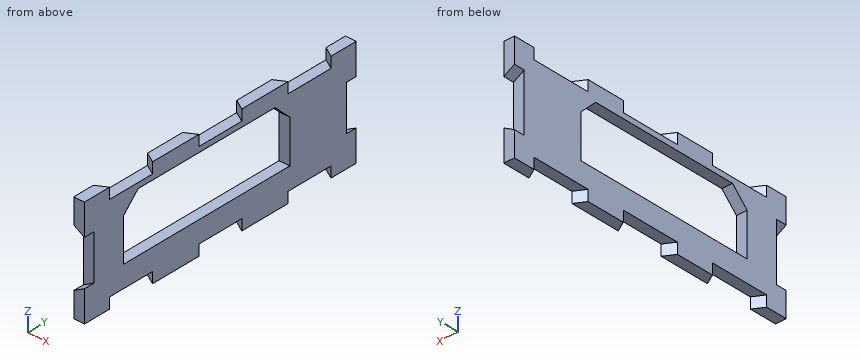
from build123d import *

# Parameters (mm, degrees)
SKETCH2_W           = 139
SKETCH2_H           = 50
BOSS_EXTRUDE1_DEPTH = 5
CUT_EXTRUDE1_DEPTH  = 5
CUT_EXTRUDE2_START  = -45
CUT_EXTRUDE2_DEPTH  = 5
CUT_EXTRUDE3_DEPTH  = 5
CUT_EXTRUDE5_START  = -134
CUT_EXTRUDE5_DEPTH  = 5
CUT_EXTRUDE6_DEPTH  = 5


with BuildPart() as part:
    # Sketch2 → Boss-Extrude1 (new body)
    with BuildSketch(Plane.YZ):
        Rectangle(SKETCH2_W, SKETCH2_H)
    extrude(amount=BOSS_EXTRUDE1_DEPTH)

    # Sketch3 → Cut-Extrude1 (cut)
    with BuildSketch(Plane(origin=(0, 0, -25), x_dir=(1, 0, 0), z_dir=(0, 0, -1))):
        Polygon((0, 31.787187079), (0, 59.5), (24, 45.643593539), align=None)
        Polygon((0, -13.856406461), (0, 13.856406461), (24, 0), align=None)
        Polygon((0, -59.5), (0, -31.787187079), (24, -45.643593539), align=None)
    extrude(amount=-CUT_EXTRUDE1_DEPTH, mode=Mode.SUBTRACT)

    # Sketch3<3> → Cut-Extrude2 (cut)
    with BuildSketch(Plane(origin=(0, 0, -25), x_dir=(1, 0, 0), z_dir=(0, 0, -1)).offset(CUT_EXTRUDE2_START)):
        Polygon((0, 31.787187079), (0, 59.5), (24, 45.643593539), align=None)
        Polygon((0, -13.856406461), (0, 13.856406461), (24, 0), align=None)
        Polygon((0, -59.5), (0, -31.787187079), (24, -45.643593539), align=None)
    extrude(amount=-CUT_EXTRUDE2_DEPTH, mode=Mode.SUBTRACT)

    # Sketch6 → Cut-Extrude3 (cut)
    with BuildSketch(Plane(origin=(0, 69.5, 0), x_dir=(-1, 0, 0), z_dir=(0, 1, 0))):
        Polygon((0, 13.423393759), (0, -13.423393759), (-23.25, 0), align=None)
    extrude(amount=-CUT_EXTRUDE3_DEPTH, mode=Mode.SUBTRACT)

    # Sketch6<3> → Cut-Extrude5 (cut)
    with BuildSketch(Plane(origin=(0, 69.5, 0), x_dir=(-1, 0, 0), z_dir=(0, 1, 0)).offset(CUT_EXTRUDE5_START)):
        Polygon((0, 13.423393759), (0, -13.423393759), (-23.25, 0), align=None)
    extrude(amount=-CUT_EXTRUDE5_DEPTH, mode=Mode.SUBTRACT)

    # Sketch4 → Cut-Extrude6 (cut)
    with BuildSketch(Plane(origin=(0, 0, 0), x_dir=(0, -1, 0), z_dir=(-1, 0, 0))):
        Polygon((-35.5, -10), (49.5, -10), (49.5, 10), (42, 17.5), (-28, 17.5), (-35.5, 10), align=None)
    extrude(amount=-CUT_EXTRUDE6_DEPTH, mode=Mode.SUBTRACT)


solid = part.part
The model under review builds one solid part; all positions refer to its coordinate system, in mm. Round coordinates to 2 decimals unless told otherwise and drop trailing zeros. Loops run counter-clockwise (first coordinate to the right, second up) from the corner with the lowest first, then second, coordinate; pieces in that order, holes last. Notation, with made-up numbers: (-30.75, -26.5) -> (-5.75, -26.5) arc R25 cw to (-5.75, -14.5) -> close; hole circle Ø11 at (28.5, -19). An arc over 180 degrees is marked (long way). Write item = value, one per line. Start each with the question number.
Item 1: Take a section at B-B on y = -40. Give the boundary of the cut face in (x, z), plus the area to 3 significant figures.
Item 2: Insertion check: pin 1 (2.5 mm diameter, centred on x = 1.5, y = -6, fed in from -Z); pin 2 (2.5 mm diameter, centred on x = 2.5, z = -2.5, fed in from -Y); pin 3 (1.5 mm diameter, centred on x = 3.5, y = -43.5, fed in from +Z). Each pin has a flat end and moves straight along its axis. Give the tip position at first contact, or say it passes through.
Item 3: Take a section at D-D on z = -12. Give the boundary of the cut face in (x, y).
Item 4: Take a section at C-C on y = 50. Give the boundary of the cut face in (x, z).
Item 5: To check wall thickness, follow L1, parallel to Y at x = 4, z = 5; L2, parallel to Z at x = 2.65, y = -19; L3, parallel to Z at x = 3.6, y = -1. State the ranges of each line that lie inside material, in increasing order.
Item 6: Take a section at A-A on z = -3. Give the boundary of the cut face in (x, y), plus the area to 3 significant figures.
Result:
q1.outline = (0, -20) -> (5, -20) -> (5, -10) -> (0, -10) -> close; (0, 17.5) -> (5, 17.5) -> (5, 20) -> (0, 20) -> close
q1.area = 62.5 mm²
q2.pin_1 = -20
q2.pin_2 = -64.5
q2.pin_3 = 20
q3.outline = (0, -64.5) -> (2.47, -64.5) -> (2.47, -69.5) -> (5, -69.5) -> (5, 69.5) -> (2.47, 69.5) -> (2.47, 64.5) -> (0, 64.5) -> close
q4.outline = (0, -20) -> (5, -20) -> (5, 20) -> (0, 20) -> close
q5.L1 = -64.5 to -49.5, 35.5 to 64.5
q5.L2 = -25 to -10, 17.5 to 25
q5.L3 = -20 to -10, 17.5 to 20
q6.outline = (0, -64.5) -> (5, -64.5) -> (5, -49.5) -> (0, -49.5) -> close; (0, 35.5) -> (5, 35.5) -> (5, 64.5) -> (0, 64.5) -> close
q6.area = 220 mm²
